For this review, take the finished solid that the model builds, in its own axes (mm). A direction names the side the tool comes from. Round coordinates to 2 decimals unless told otherwise and drop trailing zeros. Write each loop counter-clockwise with the first axis right and the second up, starting at its lowest first coordinate (ties: lowest second). Pieces come first, ordered by that corner, then holes.
from build123d import *

# Parameters (mm, degrees)
SKETCH2_R           = 2.499965
SKETCH2_R_2         = 2.49997
SKETCH2_R_3         = 2.4999655
SKETCH2_R_4         = 2.499962807
SKETCH2_R_5         = 2.4999705
SKETCH2_R_6         = 2.499967809
SKETCH2_R_7         = 2.499966
SKETCH2_R_8         = 2.4999665
SKETCH2_R_9         = 2.499966488
BOSS_EXTRUDE1_DEPTH = 9
CUT_EXTRUDE1_DEPTH  = 10
CUT_EXTRUDE2_DEPTH  = 244.998875453
SKETCH5_R           = 2.5
CUT_EXTRUDE3_DEPTH  = 244.998875453
CUT_EXTRUDE5_DEPTH  = 10
FILLET1_R           = 10


with BuildPart() as part:
    # Sketch2 → Boss-Extrude1 (new body)
    with BuildSketch(Plane.XY):
        Polygon((-211.70586, -139.55845), (122.983766, -139.55845), (211.70583, 139.558464), (-211.70586, 139.558464), align=None)
        with Locations((-192.444718, -125.900476)):
            Circle(SKETCH2_R, mode=Mode.SUBTRACT)
        with Locations((-181.028235, -121.988219)):
            Circle(SKETCH2_R_2, mode=Mode.SUBTRACT)
        with Locations((-192.0409685, -80.3042345)):
            Circle(SKETCH2_R_3, mode=Mode.SUBTRACT)
        with Locations((-179.0281635, -75.623296193)):
            Circle(SKETCH2_R_4, mode=Mode.SUBTRACT)
        with Locations((-92.3000565, -128.9494755)):
            Circle(SKETCH2_R_5, mode=Mode.SUBTRACT)
        with Locations((-76.832143809, -128.336904809)):
            Circle(SKETCH2_R_6, mode=Mode.SUBTRACT)
        with Locations((-87.928392809, -81.863553809)):
            Circle(SKETCH2_R_6, mode=Mode.SUBTRACT)
        with Locations((-75.718345809, -81.250965809)):
            Circle(SKETCH2_R_6, mode=Mode.SUBTRACT)
        with Locations((-45.325502, -86.123854)):
            Circle(SKETCH2_R, mode=Mode.SUBTRACT)
        with Locations((-21.323083, -93.781229)):
            Circle(SKETCH2_R_7, mode=Mode.SUBTRACT)
        with Locations((54.304011, -89.994307)):
            Circle(SKETCH2_R_7, mode=Mode.SUBTRACT)
        with Locations((78.1115035, -95.7303835)):
            Circle(SKETCH2_R_8, mode=Mode.SUBTRACT)
        with Locations((114.776659, 36.09363)):
            Circle(SKETCH2_R, mode=Mode.SUBTRACT)
        with Locations((86.96623, 12.266557)):
            Circle(SKETCH2_R_7, mode=Mode.SUBTRACT)
        with Locations((59.4275, 17.097677)):
            Circle(SKETCH2_R, mode=Mode.SUBTRACT)
        with Locations((-40.842451, 21.163049)):
            Circle(SKETCH2_R, mode=Mode.SUBTRACT)
        with Locations((-15.2807135, 15.9838705)):
            Circle(SKETCH2_R_8, mode=Mode.SUBTRACT)
        with Locations((32.626661, 62.749598)):
            Circle(SKETCH2_R_7, mode=Mode.SUBTRACT)
        with Locations((118.780878488, 104.469667)):
            Circle(SKETCH2_R_9, mode=Mode.SUBTRACT)
        with Locations((32.7798015, 116.8664005)):
            Circle(SKETCH2_R_8, mode=Mode.SUBTRACT)
    extrude(amount=BOSS_EXTRUDE1_DEPTH)

    # Sketch3 → Cut-Extrude1 (cut)
    with BuildSketch(Plane.XY.offset(9)):
        Polygon((147.113293383, 124.3664005), (73.705987484, -139.55845), (211.70583, -139.55845), (211.70583, 139.558464), (-211.70586, 139.558464), (-211.70586, -139.55845), (-199.944718, -139.55845), (-199.944718, -77.260214262), (29.956914073, 124.3664005), align=None)
    extrude(amount=-CUT_EXTRUDE1_DEPTH, mode=Mode.SUBTRACT)

    # Sketch4 → Cut-Extrude2 (cut, through all)
    with BuildSketch(Plane.XY.offset(9)):
        Polygon((-163.885127, -139.55845), (-147.880898, -123.554221), (-123.333708966, -123.554221), (-107.329479966, -139.55845), align=None)
    extrude(amount=-CUT_EXTRUDE2_DEPTH, mode=Mode.SUBTRACT)

    # Sketch5 → Cut-Extrude3 (cut, through all)
    with BuildSketch(Plane.XY.offset(9)):
        with Locations((-123.130898, -113.554221)):
            Circle(SKETCH5_R)
        with Locations((-78.130898, -113.554221)):
            Circle(SKETCH5_R)
        with Locations((-123.380898, -67.554221)):
            Circle(SKETCH5_R)
        with Locations((-78.130898, -67.554221)):
            Circle(SKETCH5_R)
    extrude(amount=-CUT_EXTRUDE3_DEPTH, mode=Mode.SUBTRACT)

    # Sketch6 → Cut-Extrude5 (cut)
    with BuildSketch(Plane.XY.offset(9)):
        with BuildLine():
            Line((-195.525508542, -73.384512142), (-194.933621691, -73.384512142))
            ThreePointArc((-194.933621691, -73.384512142), (-115.656074248, -30.741284252), (-46.149790694, 26.462307945))
            ThreePointArc((-46.149790694, 26.462307945), (-6.887258575, 71.211725192), (26.296691523, 120.637247226))
            Line((26.296691523, 120.637247226), (26.296691523, 121.156339417))
            Line((26.296691523, 121.156339417), (-195.525508542, -73.384512142))
        make_face()
        Polygon((147.113293383, 35.655168177), (147.113293383, 124.3664005), (122.439403996, 35.655168177), align=None)
        Polygon((-75.287663516, -135.676154132), (-93.736030822, -139.55845), (73.705987484, -139.55845), (83.854883116, -103.069632849), (79.655983667, -103.069632849), align=None)
        with BuildLine():
            Line((79.655983667, -103.069632849), (83.854883116, -103.069632849))
            Line((83.854883116, -103.069632849), (85.337218021, -97.740122205))
            ThreePointArc((85.337218021, -97.740122205), (83.24278011, -101.200301265), (79.655983667, -103.069632849))
        make_face()
        with BuildLine():
            ThreePointArc((-196.986177186, -74.665536862), (-196.011897332, -73.941709513), (-194.933621691, -73.384512142))
            Line((-194.933621691, -73.384512142), (-195.525508542, -73.384512142))
            Line((-195.525508542, -73.384512142), (-196.986177186, -74.665536862))
        make_face()
        Polygon((26.296691523, 124.3664005), (26.296691523, 121.156339417), (27.834592626, 122.505097973), (29.956914073, 124.3664005), align=None)
        with BuildLine():
            Line((27.834592626, 122.505097973), (26.296691523, 121.156339417))
            Line((26.296691523, 121.156339417), (26.296691523, 120.637247226))
            ThreePointArc((26.296691523, 120.637247226), (26.989824424, 121.633597313), (27.834592626, 122.505097973))
        make_face()
        with BuildLine():
            Line((29.956914073, 124.3664005), (27.834592626, 122.505097973))
            ThreePointArc((27.834592626, 122.505097973), (30.137854408, 123.885667952), (32.779801516, 124.3664005))
            Line((32.779801516, 124.3664005), (29.956914073, 124.3664005))
        make_face()
        with BuildLine():
            Line((147.113293383, 124.3664005), (32.779801516, 124.3664005))
            ThreePointArc((32.779801516, 124.3664005), (33.31619378, 124.347194798), (33.849838899, 124.289676055))
            Line((33.849838899, 124.289676055), (119.850915887, 111.892942555))
            ThreePointArc((119.850915887, 111.892942555), (124.449885477, 109.380100764), (126.280878488, 104.469667))
            ThreePointArc((126.280878488, 104.469667), (126.277670913, 104.250342289), (126.268050933, 104.031205177))
            Line((126.268050933, 104.031205177), (122.263831446, 35.655168177))
            Line((122.263831446, 35.655168177), (122.439403996, 35.655168177))
            Line((122.439403996, 35.655168177), (147.113293383, 124.3664005))
        make_face()
        with BuildLine():
            Line((122.002373456, 34.083891063), (122.439403996, 35.655168177))
            Line((122.439403996, 35.655168177), (122.263831446, 35.655168177))
            ThreePointArc((122.263831446, 35.655168177), (122.174935028, 34.862568747), (122.002373456, 34.083891063))
        make_face()
    extrude(amount=-CUT_EXTRUDE5_DEPTH, mode=Mode.SUBTRACT)

    # Fillet1
    # the kernel refuses this fillet: 10 mm, written as the material it adds along each edge
    with BuildSketch(Plane(origin=(-147.880898, -123.554221, 9), x_dir=(1, 0, 0), z_dir=(0, 0, -1)), Plane(origin=(-123.333708966, -123.554221, 9), x_dir=(0.707106781186551, -0.7071067811865441, 0), z_dir=(0, 0, -1))) as fillet1_piece_1:
        with BuildLine():
            CenterArc((FILLET1_R * 0.414213562373, FILLET1_R), FILLET1_R, 225, 45)
            Line((-FILLET1_R * 0.292893218813, FILLET1_R * 0.292893218813), (0, 0))
            Line((0, 0), (FILLET1_R * 0.414213562373, 0))
        make_face()
    extrude(amount=9)
    # the kernel refuses this fillet: 10 mm, written as the material it takes off along each edge
    with BuildSketch(Plane(origin=(-199.944718, -77.260214262, 20.264688934), x_dir=(0, -1, 0), z_dir=(0, 0, -1))) as fillet1_2_piece_1:
        with BuildLine():
            CenterArc((4.505875574, -10), FILLET1_R, 90, 45.239414653)
            Line((-2.5946774, -2.958540814), (0, 0))
            Line((0, 0), (4.505875574, 0))
        make_face()
    extrude(amount=31.529377868, mode=Mode.SUBTRACT)
    with BuildSketch(Plane(origin=(-163.885127, -139.55845, 19.355339059), x_dir=(-1, 0, 0), z_dir=(0, 0, -1)), Plane(origin=(-107.329479966, -139.55845, 19.355339059), x_dir=(-0.707106781186551, 0.7071067811865441, 0), z_dir=(0, 0, -1))) as fillet1_2_piece_2:
        with BuildLine():
            CenterArc((FILLET1_R * 0.414213562373, FILLET1_R), FILLET1_R, 225, 45)
            Line((-FILLET1_R * 0.292893218813, FILLET1_R * 0.292893218813), (0, 0))
            Line((0, 0), (FILLET1_R * 0.414213562373, 0))
        make_face()
    extrude(amount=29.710678119, mode=Mode.SUBTRACT)
    with BuildSketch(Plane(origin=(-93.736030822, -139.55845, 11.602018692), x_dir=(-1, 0, 0), z_dir=(0, 0, -1))) as fillet1_2_piece_3:
        with BuildLine():
            CenterArc((FILLET1_R * 0.104080747675, FILLET1_R), FILLET1_R, 258.116013885, 11.883986115)
            Line((-FILLET1_R * 0.101849941288, FILLET1_R * 0.0214334200765), (0, 0))
            Line((0, 0), (FILLET1_R * 0.104080747675, 0))
        make_face()
    extrude(amount=14.204037384, mode=Mode.SUBTRACT)
    with BuildSketch(Plane(origin=(-199.944718, -139.55845, 34), x_dir=(1, 0, 0), z_dir=(0, 0, -1))) as fillet1_2_piece_4:
        with BuildLine():
            CenterArc((FILLET1_R, -FILLET1_R), FILLET1_R, 90, 90)
            Line((0, -FILLET1_R), (0, 0))
            Line((0, 0), (FILLET1_R, 0))
        make_face()
    extrude(amount=59, mode=Mode.SUBTRACT)


solid = part.part
(1) For faces 4 (the face through (2, -39, 0)), 5 (the face through (-147.62, -124.34, 4.56)), list the 3-axis set-ups (+Z, -Z, +X, -X, +Y, -Y) from which the entire face can be reached by the end or side of a thin tool; tool diameter is ignored.
Geometry check:
face 4: -Z, +X, -X, +Y, -Y
face 5: +Z, -Z, -Y
(2) We need section A-A, the plane x = 96.5. Give the boundary of the cut face in (y, z).
Geometry check:
outline: (-57.61, 0) - (115.26, 0) - (115.26, 9) - (-57.61, 9) - close
(3) We need section B-B, the plane z = 5. State how many separate pieces and enclosed holes the cut face has, and give its area (3 significant figures).
Geometry check:
separate pieces: 1
enclosed holes: 24
area: 48,100 mm2
(4) Mouldability with a two-part tool opening along X and no side actions: class faces 1 (the face through (-136, -123.554, 5)), 2 (the face through (-199.197, -77.971, 4.563)), 3 (the face through (124.294, 70.322, 4.563)) as pulls with the +X half, pulls with the -X half, needs draft (parallel to the pull), parting line crosses it, or undercut.
Geometry check:
face 1: undercut
face 2: pulls with the -X half
face 3: pulls with the +X half
(5) For pin 1 Ø1 at (y, z) = (-80.5, 5) entering from +X; pin 2 Ø1 at (y, z) = (-61.5, 5.5) entering from -X; pin 3 Ø1 at (x, z) = (51.5, 5.5) entering from +Y, all flat-tipped, find the tip position at first contact; note any pin that passes through.
Geometry check:
pin 1: stops at x = 90.27
pin 2: stops at x = -169.83
pin 3: stops at y = 121.82
(6) We need section C-C, the plane y = -59.5. Give the boundary of the cut face in (x, z).
Geometry check:
outline: (-164.81, 0) - (95.97, 0) - (95.97, 9) - (-164.81, 9) - close
(7) For line 1 along Y through (x, z) = (58.5, 4.5); line 2 along X through (y, z) = (63, 4.25); line 3 along X through (y, z) = (-93, 4.75), list the stretches that pass through material, from the lowest coordinate up.
Geometry check:
line 1: y = -107.52 to 14.78, 19.42 to 120.74
line 2: x = -13.35 to 30.14, 35.11 to 123.87
line 3: x = -199.94 to -23.7, -18.95 to 86.66
